```python
from build123d import *

# Parameters (mm, degrees)
F0_W     = 152.4
F0_H     = 114.3
F1_DEPTH = 6.35
F2_R     = 9.525
F3_DEPTH = 25.4
F5_R     = 12.7
F6_W     = 50.8
F6_H     = 6.35
F7_DEPTH = 25.4


with BuildPart() as f1:
    # F0 (on Top) → F1 (new body)
    with BuildSketch(Plane.XY):
        Rectangle(F0_W, F0_H)
    extrude(amount=F1_DEPTH)

    # F2 (on face) → F3 (cut)
    with BuildSketch(Plane(origin=(0, 0, 0), x_dir=(1, 0, 0), z_dir=(0, 0, -1))):
        with Locations((-38.1, 0)):
            Circle(F2_R)
        with Locations((-38.1, 31.75)):
            Circle(F2_R)
        with Locations((-38.1, -31.75)):
            Circle(F2_R)
    extrude(amount=-F3_DEPTH, mode=Mode.SUBTRACT)

    # F5
    f5_edges = [f1.edges().sort_by_distance(p)[0] for p in [
        (-76.2, -57.15, 3.175),
        (-76.2, 57.15, 3.175),
        (76.2, 57.15, 3.175),
        (76.2, -57.15, 3.175),
    ]]
    fillet(f5_edges, radius=F5_R)

    # F6 (on face) → F7 (cut)
    with BuildSketch(Plane(origin=(0, 0, 0), x_dir=(1, 0, 0), z_dir=(0, 0, -1))):
        with Locations((38.1, -41.275)):
            Rectangle(F6_W, F6_H)
    extrude(amount=-F7_DEPTH, mode=Mode.SUBTRACT)


solid = f1.part
```
Verification items for the finished model (mm, model axes). A direction names the side the tool comes from. Give positions to 0.01 mm unless a question says otherwise; leave off trailing zeros. Order: outer loops, then holes, each group sorted by start corner. A loop starts at its lowest first (then second) coordinate and runs counter-clockwise, first axis right, second up. Notation, with made-up numbers: M 51.25,42 L 87.25,42 A22 ccw 87.25,62 Z; hole C 85,-32.75 d5. An arc over 180 degrees is marked long. Return JSON: item names as keys, results as strings. Group by question number.
1) Section check A-A on x = 30. Record the cut outline in (y, z), and give its area (3 significant figures).
2) Scan lines: line 1 (Y direction, x = -38, z = 2.5); line 2 (Y direction, x = -34, z = 5.75); line 3 (Y direction, x = 23.5, z = 2). Record each from-to range of solid material in increasing order.
3) Access from +Z, -Z, +X, -X, +Y, -Y to the whole of each face (thin tool, end or side, straight path). Record for faces 4 (the face through (76.2, -1, 3)), 5 (the face through (12.7, 41, 3)).
4) Section check B-B on y = -31.75. Record the cut outline in (x, z) (3 decimals).
5) Section check D-D on z = 4.5. Record the cut outline in (x, y) (3 decimals), and give its area (3 significant figures).
6) Mould release check, pull along Y, two halves, no side actions. Record for faces 1 (the face through (-1, 57.15, 3)), 2 (the face through (-33.7, 40.2, 3.1)), 3 (the face through (-72.58, -53.33, 3.22)): pulls with the +Y half, pulls with the -Y half, needs draft (parallel to the pull), parting line crosses it, or undercut.
7) Section check C-C on x = -38.1. Record the cut outline in (y, z) (3 decimals).
8) Go/stop test with a flat-tipped pin: pin 1 Ø17 at (x, y) = (-38.1, 0) entering from -Z. Record where the tip stops, or that it passes through.
Answer block:
{
 "1": {"outline": "M -57.15,0 L 38.1,0 L 38.1,6.35 L -57.15,6.35 Z; M 44.45,0 L 57.15,0 L 57.15,6.35 L 44.45,6.35 Z", "area": "685 mm^2"},
 "2": {"line 1": "y = -57.15 to -41.27, -22.23 to -9.52, 9.52 to 22.23, 41.27 to 57.15", "line 2": "y = -57.15 to -40.35, -23.15 to -8.6, 8.6 to 23.15, 40.35 to 57.15", "line 3": "y = -57.15 to 38.1, 44.45 to 57.15"},
 "3": {"face 4": "+Z, -Z, +X, +Y, -Y", "face 5": "+Z, -Z"},
 "4": {"outline": "M -76.2,0 L -47.625,0 L -47.625,6.35 L -76.2,6.35 Z; M -28.575,0 L 76.2,0 L 76.2,6.35 L -28.575,6.35 Z"},
 "5": {"outline": "M -76.2,-44.45 A12.7 ccw -63.5,-57.15 L 63.5,-57.15 A12.7 ccw 76.2,-44.45 L 76.2,44.45 A12.7 ccw 63.5,57.15 L -63.5,57.15 A12.7 ccw -76.2,44.45 Z; hole C -38.1,-31.75 d19.05; hole C -38.1,0 d19.05; hole C -38.1,31.75 d19.05; hole M 12.7,38.1 L 63.5,38.1 L 63.5,44.45 L 12.7,44.45 Z", "area": "16,100 mm^2"},
 "6": {"face 1": "pulls with the +Y half", "face 2": "undercut", "face 3": "pulls with the -Y half"},
 "7": {"outline": "M -57.15,0 L -41.275,0 L -41.275,6.35 L -57.15,6.35 Z; M -22.225,0 L -9.525,0 L -9.525,6.35 L -22.225,6.35 Z; M 9.525,0 L 22.225,0 L 22.225,6.35 L 9.525,6.35 Z; M 41.275,0 L 57.15,0 L 57.15,6.35 L 41.275,6.35 Z"},
 "8": {"pin 1": "passes through"}
}
